Read the model definition and answer for the solid it produces. Units are mm, in the model's axes. Face numbers are marked on the shaded views. A direction names the side the tool comes from. Coordinates: 2 decimals unless noted, no trailing zeros. Loops run counter-clockwise (first coordinate to the right, second up) from the corner with the lowest first, then second, coordinate; pieces in that order, holes last.
from build123d import *

# Parameters (mm, degrees)
F0_W           = 78.25
F0_H           = 40
F1_DEPTH       = 23.1
F2_W           = 76.25
F2_H           = 36
F3_DEPTH       = 21.1
F5_D           = 11
F5_DEPTH       = 10
F5_CBORE_D     = 12
F5_CBORE_DEPTH = 1
F7_W           = 21
F7_H           = 19
F8_DEPTH       = 25.4
F8_DEPTH_BACK  = 25.4


with BuildPart() as f1:
    # F0 (on Top) → F1 (new body)
    with BuildSketch(Plane.XY):
        Rectangle(F0_W, F0_H)
    extrude(amount=F1_DEPTH)

    # F2 (on face) → F3 (cut)
    with BuildSketch(Plane.XY.offset(23.1)):
        Rectangle(F2_W, F2_H)
    extrude(amount=-F3_DEPTH, mode=Mode.SUBTRACT)

    # F5
    with Locations(Plane(origin=(0, -18, 0), x_dir=(-1, 0, 0), z_dir=(0, 1, 0))):
        with Locations((32.125, 16.76)):
            CounterBoreHole(F5_D / 2, F5_CBORE_D / 2, F5_CBORE_DEPTH, depth=F5_DEPTH)

    # F7 (on face) → F8 (cut, two sides)
    with BuildSketch(Plane.XZ.offset(-18)) as f8_sk:
        with Locations((0, 12.55)):
            Rectangle(F7_W, F7_H)
    extrude(amount=-F8_DEPTH, mode=Mode.SUBTRACT)
    extrude(f8_sk.sketch, amount=-F8_DEPTH_BACK, mode=Mode.SUBTRACT)


solid = f1.part
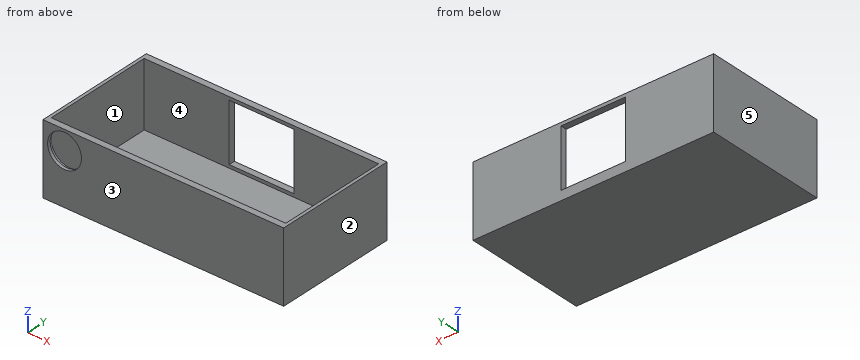
Item 1: A cutting plane is placed at D-D on z = 20.5. Determine the outline of the cut face in (x, y) (3 decimals).
Numbers:
outline: (-39.125, -20) - (-36.158, -20) - (-36.158, -19) - (-36.817, -19) - (-36.817, -18) - (-38.125, -18) - (-38.125, 18) - (-10.5, 18) - (-10.5, 20) - (-39.125, 20) - close; (-28.092, -20) - (39.125, -20) - (39.125, 20) - (10.5, 20) - (10.5, 18) - (38.125, 18) - (38.125, -18) - (-27.433, -18) - (-27.433, -19) - (-28.092, -19) - close
Item 2: A cutting plane is placed at B-B on z = 15.5. Determine the outline of the cut face in (x, y) (3 decimals), then the cut area to 3 significant figures.
Numbers:
outline: (-39.125, -20) - (-37.479, -20) - (-37.479, -19) - (-37.991, -19) - (-37.991, -18) - (-38.125, -18) - (-38.125, 18) - (-10.5, 18) - (-10.5, 20) - (-39.125, 20) - close; (-26.771, -20) - (39.125, -20) - (39.125, 20) - (10.5, 20) - (10.5, 18) - (38.125, 18) - (38.125, -18) - (-26.259, -18) - (-26.259, -19) - (-26.771, -19) - close
area: 321 mm2
Item 3: Find the intervals of material crossed by line 1 along Y through (x, z) = (27, 7.25); line 2 along X through (y, z) = (-3.5, 12.75) (3 decimals); line 3 along Z through (x, y) = (35.5, -3), in increasing order.
Numbers:
line 1: y = -20 to -18, 18 to 20
line 2: x = -39.125 to -38.125, 38.125 to 39.125
line 3: z = 0 to 2
Item 4: A cutting plane is placed at C-C on y = -12. Determine the outline of the cut face in (x, z) (3 decimals).
Numbers:
outline: (-39.125, 0) - (39.125, 0) - (39.125, 23.1) - (38.125, 23.1) - (38.125, 2) - (-38.125, 2) - (-38.125, 23.1) - (-39.125, 23.1) - close
Item 5: A cutting plane is placed at A-A on x = 9. Determine the outline of the cut face in (y, z), then the cut area to 3 significant figures.
Numbers:
outline: (-20, 0) - (20, 0) - (20, 3.05) - (18, 3.05) - (18, 2) - (-18, 2) - (-18, 23.1) - (-20, 23.1) - close; (18, 22.05) - (20, 22.05) - (20, 23.1) - (18, 23.1) - close
area: 126 mm2
Item 6: Determine the mould class of the marked faces 3, 4 and 5 for opening direction X: released by +X, released by -X, zero draft, split by the parting line, or undercut.
Numbers:
face 3: zero draft
face 4: undercut
face 5: released by -X
Item 7: Given pin 1 (10 mm diameter, centred on x = 17.5, y = -11, fed in from +Z); pin 2 (2 mm diameter, centred on x = 2, z = 13, fed in from +Y); pin 3 (1 mm diameter, centred on x = 2, y = 19, fed in from -Z), each flat-ended and moving along its own axis, determine where each tip first touches the part or whether it passes through.
Numbers:
pin 1: stops at z = 2
pin 2: stops at y = -18
pin 3: stops at z = 0
Item 8: Which of the six approach directions +Z, -Z, +X, -X, +Y, -Y give full straight-line access (tool end or side, diameter ignored) to the marked faces 1 and 2?
Numbers:
face 1: +Z
face 2: +Z, -Z, +X, +Y, -Y
